from build123d import *

# Parameters (mm, degrees)
SKETCH1_R           = 0.425
SKETCH1_R_2         = 0.8
BOSS_EXTRUDE1_DEPTH = 1.6
CUT_EXTRUDE1_DEPTH  = 0.0001
CUT_EXTRUDE2_DEPTH  = 0.0001
PARTFOOTPRINTS_W    = 30.48
PARTFOOTPRINTS_H    = 7.989227112
PARTFOOTPRINTS_W_2  = 3.5
PARTFOOTPRINTS_H_2  = 6.95
CUT_EXTRUDE3_DEPTH  = 0.0001
CUT_EXTRUDE4_DEPTH  = 2.6
SKETCH3_W           = 7.779754111
SKETCH3_H           = 5.155241991
CUT_EXTRUDE5_DEPTH  = 10
FILLET1_R           = 1
CUT_EXTRUDE6_DEPTH  = 2.6
FILLET2_R           = 1
SKETCH5_R           = 1.125
CUT_EXTRUDE7_DEPTH  = 2.6
SKETCH6_R           = 1.2
CUT_EXTRUDE8_DEPTH  = 2.6


with BuildPart() as part:
    # Sketch1 → Boss-Extrude1 (new body)
    with BuildSketch(Plane(origin=(0, 0, -0.0125), x_dir=(-1, 0, 0), z_dir=(0, 0, -1))):
        with BuildLine():
            Line((35.3, -50), (35.3, -48))
            ThreePointArc((35.3, -48), (35.592893219, -47.292893219), (36.3, -47))
            Line((36.3, -47), (45.8, -47))
            ThreePointArc((45.8, -47), (46.507106781, -46.707106781), (46.8, -46))
            Line((46.8, -46), (46.8, -41.4))
            ThreePointArc((46.8, -41.4), (47.092893219, -40.692893219), (47.8, -40.4))
            Line((47.8, -40.4), (49.3, -40.4))
            Line((49.3, -40.4), (49.3, 39.2))
            Line((49.3, 39.2), (43.2, 45.3))
            Line((43.2, 45.3), (35.500000002, 45.3))
            Line((35.500000002, 45.3), (35.500000002, 43.8))
            ThreePointArc((35.500000002, 43.8), (35.207106783, 43.092893219), (34.500000002, 42.8))
            Line((34.500000002, 42.8), (4.499999998, 42.8))
            ThreePointArc((4.499999998, 42.8), (3.792893217, 43.092893219), (3.499999998, 43.8))
            Line((3.499999998, 43.8), (3.499999998, 45.3))
            Line((3.499999998, 45.3), (-43.2, 45.3))
            Line((-43.2, 45.3), (-49.3, 39.2))
            Line((-49.3, 39.2), (-49.3, -40.4))
            Line((-49.3, -40.4), (-47.8, -40.4))
            ThreePointArc((-47.8, -40.4), (-47.092893219, -40.692893219), (-46.8, -41.4))
            Line((-46.8, -41.4), (-46.8, -46))
            ThreePointArc((-46.8, -46), (-46.507106781, -46.707106781), (-45.8, -47))
            Line((-45.8, -47), (-36.3, -47))
            ThreePointArc((-36.3, -47), (-35.592893219, -47.292893219), (-35.3, -48))
            Line((-35.3, -48), (-35.3, -50))
            Line((-35.3, -50), (35.3, -50))
        make_face()
        with Locations((-21.27, 41.37)):
            Circle(SKETCH1_R, mode=Mode.SUBTRACT)
        with Locations((-23.81, 41.37)):
            Circle(SKETCH1_R, mode=Mode.SUBTRACT)
        with Locations((-22.54, 40.1)):
            Circle(SKETCH1_R, mode=Mode.SUBTRACT)
        with Locations((-13.87, 41.37)):
            Circle(SKETCH1_R, mode=Mode.SUBTRACT)
        with Locations((-23.81, 38.83)):
            Circle(SKETCH1_R, mode=Mode.SUBTRACT)
        with Locations((-16.41, 41.37)):
            Circle(SKETCH1_R, mode=Mode.SUBTRACT)
        with Locations((-15.14, 40.1)):
            Circle(SKETCH1_R, mode=Mode.SUBTRACT)
        with Locations((-21.27, 38.83)):
            Circle(SKETCH1_R, mode=Mode.SUBTRACT)
        with Locations((-28.67, 41.37)):
            Circle(SKETCH1_R, mode=Mode.SUBTRACT)
        with Locations((-31.21, 41.37)):
            Circle(SKETCH1_R, mode=Mode.SUBTRACT)
        with Locations((-16.41, 38.83)):
            Circle(SKETCH1_R, mode=Mode.SUBTRACT)
        with Locations((-29.94, 40.1)):
            Circle(SKETCH1_R, mode=Mode.SUBTRACT)
        with Locations((-31.21, 38.83)):
            Circle(SKETCH1_R, mode=Mode.SUBTRACT)
        with Locations((-28.67, 38.83)):
            Circle(SKETCH1_R, mode=Mode.SUBTRACT)
        with Locations((33.775, 38.54)):
            Circle(SKETCH1_R_2, mode=Mode.SUBTRACT)
        with Locations((5.225, 38.54)):
            Circle(SKETCH1_R_2, mode=Mode.SUBTRACT)
        with Locations((-13.87, 38.83)):
            Circle(SKETCH1_R, mode=Mode.SUBTRACT)
    extrude(amount=-BOSS_EXTRUDE1_DEPTH)

    # thermalContacts_lower → Cut-Extrude1 (cut)
    with BuildSketch(Plane(origin=(0, 0, -0.0125), x_dir=(-1, 0, 0), z_dir=(0, 0, -1))):
        Polygon((47, 35.5), (47, -41.5), (59.827263463, -41.5), (59.827263463, 48.757689229), (41.5, 48.757689229), (41.5, 41.5), (41.5, 35.5), align=None)
        Polygon((-47, 35.5), (-47, -41.5), (-56.192158269, -41.5), (-56.192158269, 47), (-41.5, 47), (-41.5, 41.5), (-41.5, 35.5), align=None)
    extrude(amount=-CUT_EXTRUDE1_DEPTH, mode=Mode.SUBTRACT)

    # thermalContacts_upper → Cut-Extrude2 (cut)
    with BuildSketch(Plane.XY.offset(1.5875)):
        Polygon((-47, 35.5), (-47, -41.5), (-56.192158269, -41.5), (-56.192158269, 47), (-41.5, 47), (-41.5, 41.5), (-41.5, 35.5), align=None)
        Polygon((47, 35.5), (47, -41.5), (59.827263463, -41.5), (59.827263463, 47), (41.5, 47), (41.5, 41.5), (41.5, 35.5), align=None)
    extrude(amount=-CUT_EXTRUDE2_DEPTH, mode=Mode.SUBTRACT)

    # partFootprints → Cut-Extrude3 (cut)
    with BuildSketch(Plane.XY.offset(1.5875)):
        with Locations((-19.5, 38.834613556)):
            Rectangle(PARTFOOTPRINTS_W, PARTFOOTPRINTS_H)
        with Locations((15.14, 41.825)):
            Rectangle(PARTFOOTPRINTS_W_2, PARTFOOTPRINTS_H_2)
        with Locations((22.54, 41.825)):
            Rectangle(PARTFOOTPRINTS_W_2, PARTFOOTPRINTS_H_2)
        with Locations((29.94, 41.825)):
            Rectangle(PARTFOOTPRINTS_W_2, PARTFOOTPRINTS_H_2)
    extrude(amount=-CUT_EXTRUDE3_DEPTH, mode=Mode.SUBTRACT)

    # Sketch2 → Cut-Extrude4 (cut, through all)
    with BuildSketch(Plane.XY.offset(1.5875)):
        with BuildLine():
            Line((29.2, -42.8), (29.2, -40.414213562))
            ThreePointArc((29.2, -40.414213562), (29.2, -39), (30.614213562, -39))
            Line((30.614213562, -39), (31.485786438, -39))
            ThreePointArc((31.485786438, -39), (32.9, -39), (32.9, -40.414213562))
            Line((32.9, -40.414213562), (32.9, -42.8))
            Line((32.9, -42.8), (36.05, -42.8))
            Line((36.05, -42.8), (36.05, -50))
            Line((36.05, -50), (26.05, -50))
            Line((26.05, -50), (26.05, -42.8))
            Line((26.05, -42.8), (29.2, -42.8))
        make_face()
    extrude(amount=-CUT_EXTRUDE4_DEPTH, mode=Mode.SUBTRACT)

    # Sketch3 → Cut-Extrude5 (cut)
    with BuildSketch(Plane.XY.offset(1.5875)):
        with Locations((35.630924609, -49.577620995)):
            Rectangle(SKETCH3_W, SKETCH3_H)
    extrude(amount=-CUT_EXTRUDE5_DEPTH, mode=Mode.SUBTRACT)

    # Fillet1
    fillet1_edges = [part.edges().sort_by_distance(p)[0] for p in [
        (26.05, -50, 0.7875),
        (26.05, -42.8, 0.7875),
        (36.05, -42.8, 0.7875),
        (36.05, -47, 0.7875),
    ]]
    fillet(fillet1_edges, radius=FILLET1_R)

    # Sketch4 → Cut-Extrude6 (cut, through all)
    with BuildSketch(Plane.XY.offset(1.5875)):
        with BuildLine():
            Line((-51.38081647, -30.3), (-44.014213562, -30.3))
            ThreePointArc((-44.014213562, -30.3), (-42.6, -30.3), (-42.6, -31.714213562))
            Line((-42.6, -31.714213562), (-42.6, -47))
            Line((-42.6, -47), (-51.38081647, -47))
            Line((-51.38081647, -47), (-51.38081647, -30.3))
        make_face()
    extrude(amount=-CUT_EXTRUDE6_DEPTH, mode=Mode.SUBTRACT)

    # Fillet2
    fillet2_edges = [part.edges().sort_by_distance(p)[0] for p in [
        (-42.6, -47, 0.7875),
    ]]
    fillet(fillet2_edges, radius=FILLET2_R)

    # Sketch5 → Cut-Extrude7 (cut, through all)
    with BuildSketch(Plane.XY.offset(1.5875)):
        with Locations((-40.175, -23.1)):
            Circle(SKETCH5_R)
        with BuildLine():
            Line((-30.525, -24.225), (-30.825, -24.225))
            ThreePointArc((-30.825, -24.225), (-31.95, -23.1), (-30.825, -21.975))
            Line((-30.825, -21.975), (-30.525, -21.975))
            ThreePointArc((-30.525, -21.975), (-29.4, -23.1), (-30.525, -24.225))
        make_face()
    extrude(amount=-CUT_EXTRUDE7_DEPTH, mode=Mode.SUBTRACT)

    # Sketch6 → Cut-Extrude8 (cut, through all)
    with BuildSketch(Plane.XY.offset(1.5875)):
        with Locations((-37.6, -40.75)):
            Circle(SKETCH6_R)
        with Locations((-37.6, -45.25)):
            Circle(SKETCH6_R)
    extrude(amount=-CUT_EXTRUDE8_DEPTH, mode=Mode.SUBTRACT)


solid = part.part
Can you work these out from the model? Positions are in its coordinate system, mm. Give positions to 0.01 mm unless a question says otherwise; leave off trailing zeros. One line per item, written item: value.
1) Imagine slicing it at A-A on z = 0.7. Count the separate pieces of the cut face and the enclosed holes in it, and give its area (3 significant figures).
Geometry check:
separate pieces: 1
enclosed holes: 21
area: 8,950 mm²
2) Please list where these lines run through material, in increasing order: line 1 (Y direction, x = 23.81, z = 1.3) (3 decimals); line 2 (Y direction, x = 29.94, z = 1.05) (3 decimals); line 3 (Y direction, x = -11.5, z = 0.3).
Geometry check:
line 1: y = -50 to 38.405, 39.255 to 40.945, 41.795 to 45.3
line 2: y = -38.708 to 39.675, 40.525 to 45.3
line 3: y = -50 to 42.8
3) I'm going to push flat-ended pins straight in: pin 1 (0.8 mm diameter, centred on y = -41.5, z = 1, fed in from +X); pin 2 (0.5 mm diameter, centred on y = -47, z = 0.5, fed in from +X); pin 3 (0.8 mm diameter, centred on y = 44.5, z = 0.5, fed in from -X). Where does each tip first touch, or does it pass through?
Geometry check:
pin 1: stops at x = 46.85
pin 2: stops at x = 46.46
pin 3: stops at x = -44.4
4) Thinking about a two-plate mould opening in X: for faces 1 (the face through (-46.3, 42.2, 0.8)), 2 (the face through (-38.484, -39.939, 0.799)), 3 (the face through (30, 42, 1.587)), which applies, +X half, -X half, draft (parallel to the pull), parting line (faces both ways), or undercut?
Geometry check:
face 1: -X half
face 2: undercut
face 3: draft
